The model under review builds one solid part; all positions refer to its coordinate system, in mm. A direction names the side the tool comes from. Coordinates: 2 decimals unless noted, no trailing zeros. Write each loop counter-clockwise with the first axis right and the second up, starting at its lowest first coordinate (ties: lowest second). Pieces come first, ordered by that corner, then holes.
1) Machinability: for faces 1 (the flat face through (-150, -308, 84)), 2 (the flat face through (-170, -318, 79)), 3 (the flat face through (-156, 150, 84)), 4 (the flat face through (170, -154, 79)), which of the approach directions +Z, -Z, +X, -X, +Y, -Y give a long, thin tool a straight path to every point of the face, cutting with its end or side? Answer none if there is none.
2) Mouldability with a two-part tool opening along X and no side actions: class faces 5 (the flat face through (-95, -87, 10)), 6 (the flat face through (-470, 26, 9)), 7 (the flat face through (-240, -167, 160)) as released by +X, released by -X, zero draft, split by the parting line, or undercut.
3) For P1, Ø3, axis at x = -262, z = 55.5, coming from the -Y side; P2, Ø5, axis at x = -117.5, y = -380, coming from the +Z side; P3, Ø12, axis at y = 80.5, z = 75, coming from the -X side; P4, Ø10, axis at x = -106.5, y = -399, coming from the -Z side, all flat-tipped, find the tip position at first contact; note any pin that passes through.
4) For line 1 (Y direction, x = -392.5, z = 92.5); line 2 (X direction, y = 29, z = 15.5), list the stretches that pass through material, from the lowest coordinate up.
5) Add section A-A, the plane z = 130. State the section outline as (x, y) points.
6) Add section B-B, the plane y = 37. State the section outline as (x, z) points, then the cut area to 3 significant figures.
Autodesk Inventor part; units mm, degrees
ref_plane "YZ Plane" through (0, 0, 0) normal (1, 0, 0) x (0, 1, 0)
ref_plane "XZ Plane" through (0, 0, 0) normal (0, 1, 0) x (-1, 0, 0)
ref_plane "XY Plane" through (0, 0, 0) normal (0, 0, 1) x (1, 0, 0)
sketch "Эскиз1" plane through (0, 0, 0) normal (0, 0, 1) x (1, 0, 0)
  line L0 (150, 150) -> (-150, 150)
  line L1 (-150, 150) -> (-150, -150)
  line L2 (-150, -150) -> (150, -150)
  line L3 (150, -150) -> (150, 150)
  line L4 (150, 150) -> (-150, -150) construction
  line L5 (-150, 150) -> (150, -150) construction
  line L6 (-450, 150) -> (-150, 150)
  line L7 (-150, 150) -> (-150, -150)
  line L8 (-150, -150) -> (-450, -150)
  line L9 (-450, -150) -> (-450, 150)
  line L10 (-450, 150) -> (-150, -150) construction
  line L11 (-150, 150) -> (-450, -150) construction
  line L12 (150, -150) -> (-150, -150)
  line L13 (-150, -150) -> (-150, -450)
  line L14 (-150, -450) -> (150, -450)
  line L15 (150, -450) -> (150, -150)
  line L16 (150, -150) -> (-150, -450) construction
  line L17 (-150, -150) -> (150, -450) construction
  line L18 (170, 170) -> (-170, 170)
  line L19 (-170, 170) -> (-170, -170)
  line L20 (-170, -170) -> (170, -170)
  line L21 (170, -170) -> (170, 170)
  line L22 (170, -130) -> (-170, -130)
  line L23 (-170, -130) -> (-170, -470)
  line L24 (-170, -470) -> (170, -470)
  line L25 (170, -470) -> (170, -130)
  line L26 (-470, -170) -> (-130, -170)
  line L27 (-130, -170) -> (-130, 170)
  line L28 (-130, 170) -> (-470, 170)
  line L29 (-470, 170) -> (-470, -170)
  point P0 (0, 0)
  point P1 (-300, 0)
  point P2 (0, -300)
  point P3 (-170, 170)
  point P4 (170, -170)
  dimension "d0" = 300
  dimension "d1" = 300
  dimension "d2" = 300
  dimension "d3" = 300
  dimension "d4" = 300
  dimension "d5" = 300
  dimension "d6" = 20
  dimension "d7" = 20
  dimension "d8" = 20
extrude "Выдавливание1" add sketch "Эскиз1" along normal blind 10
sketch "Эскиз2" plane through (0, 0, 10) normal (0, 0, 1) x (1, 0, 0)
  line L0 (170, 170) -> (-470, 170)
  line L1 (-470, 170) -> (-470, -170)
  line L2 (-470, -170) -> (-170, -170)
  line L3 (-170, -170) -> (-170, -470)
  line L4 (-170, -470) -> (170, -470)
  line L5 (170, -470) -> (170, 170)
  line L6 (150, 150) -> (-450, 150)
  line L7 (-450, 150) -> (-450, -150)
  line L8 (-450, -150) -> (-150, -150)
  line L9 (-150, -150) -> (-150, -450)
  line L10 (-150, -450) -> (150, -450)
  line L11 (150, -450) -> (150, 150)
  line L12 (-170, -470) -> (170, -470)
  line L13 (150, -450) -> (-150, -450)
  line L14 (-150, -450) -> (-150, -470)
  line L15 (-150, -470) -> (150, -470)
  line L16 (150, -470) -> (150, -450)
  line L17 (-470, 170) -> (-470, -170)
  line L18 (-450, 150) -> (-470, 150)
  line L19 (-470, 150) -> (-470, -150)
  line L20 (-470, -150) -> (-450, -150)
  line L21 (-450, -150) -> (-450, 150)
  point P0 (0, 0)
  dimension "d11" = 20
extrude "Выдавливание2" add sketch "Эскиз2" along normal blind 150 contours L5 L4 L16 L11 L6 L18 L1 L0 | L20 L8 L9 L14 L4 L3 L2 L1
sketch "Эскиз3" plane through (-470, 150, 10) normal (0, -1, 0) x (1, 0, 0)
  line L0 (620, 0) -> (0, 0)
  line L1 (620, 0) -> (620, 150)
  line L2 (0, 150) -> (620, 150)
  line L3 (0, 0) -> (0, 150)
  line L4 (620, 0) -> (620, 150)
  line L5 (620, 70) -> (0, 70)
  line L6 (0, 0) -> (0, 150)
  line L7 (620, 30) -> (0, 30)
  line L8 (620, 110) -> (0, 110)
  point P0 (470, -10)
  dimension "d14" = 70
  dimension "d15" = 40
  dimension "d16" = 40
properties part number "labik"
Geometry results:
1. face 1: +Z, -Y
1. face 2: +Z, -Z, -X, -Y
1. face 3: +Z, -X
1. face 4: +Z, -Z, +X, +Y, -Y
2. face 5: undercut
2. face 6: released by -X
2. face 7: zero draft
3. P1: stops at y = -170
3. P2: stops at z = 10
3. P3: stops at x = 150
3. P4: stops at z = 0
4. line 1: y = -170 to -150, 150 to 170
4. line 2: x = 150 to 170
5. outline: (-470, -170) - (-170, -170) - (-170, -470) - (-150, -470) - (-150, -150) - (-470, -150) - close; (-470, 150) - (150, 150) - (150, -470) - (170, -470) - (170, 170) - (-470, 170) - close
6. outline: (-470, 0) - (170, 0) - (170, 160) - (150, 160) - (150, 10) - (-470, 10) - close
6. area: 9,400 mm2
